Can you work these out from the model? Positions are in its coordinate system, mm. A direction names the side the tool comes from. Give positions to 0.01 mm unless a question says otherwise; leave off trailing zeros. Order: outer loops, then holes, each group sorted by start corner. A loop starts at its lowest first (then second) coordinate and runs counter-clockwise, first axis right, second up.
Item 1: If we mould it in two halves opening along X, with no side actions, what happens to faces 1 (the flat face through (17, 22, -10)), 2 (the cylindrical face through (-7.35, 5.1, -12.31)), 3 (the cylindrical face through (24.765, 5.028, 4.975))? For each: +X half, -X half, draft (parallel to the pull), parting line (faces both ways), or undercut.
Item 2: I want a section at A-A, the plane y = 16.75. Write out the boundary of the cut face in (x, z), then the cut area to 3 significant figures.
Item 3: I'm going to push flat-ended pins straight in: pin 1 Ø2 at (x, z) = (16, -2.5) entering from +Y; pin 2 Ø5 at (x, y) = (-6, 6.5) entering from +Z; pin 3 Ø3.5 at (y, z) = (2, 5) entering from -X. Where does each tip first touch, or does it pass through?
Item 4: If I drill on line 1 along Y through (x, z) = (-26, -17); line 2 along X through (y, z) = (8.5, 20.5); line 3 along Y through (x, z) = (6, 16), over which ranges is the centre line in solid material (lowest first)?
Item 5: Which directions (+Z, -Z, +X, -X, +Y, -Y) give clear straight access to the entire face, cutting with the end or side of a thin tool? Please do faces 4 (the flat face through (-7, 2, -13.169)), 5 (the flat face through (0, 5, -18.829)), 6 (the cylindrical face through (2.94, 15.92, 9.35)).
```python
from build123d import *

# Parameters (mm, degrees)
SALIENTE_EXTRUIR1_DEPTH    = 10
CROQUIS2_R                 = 2.5
CORTAR_EXTRUIR1_DEPTH      = 10
CROQUIS3_R                 = 9.8
SALIENTE_EXTRUIR2_DEPTH    = 12
CROQUIS4_W                 = 17.653456823
CROQUIS4_H                 = 4
CORTAR_EXTRUIR2_DEPTH      = 11.5
CORTAR_EXTRUIR3_DEPTH      = 62.373730343
CORTAR_EXTRUIR3_DEPTH_BACK = 62.373730343
CROQUIS5_W                 = 3.232473087
CROQUIS5_H                 = 4
REDONDEO1_R                = 1
REDONDEO2_R                = 5
MATRIZC7_COUNT             = 5
REDONDEO3_R                = 1
REDONDEO4_R                = 5
CORTAR_EXTRUIR4_DEPTH      = 54.438308108
CORTAR_EXTRUIR4_DEPTH_BACK = 6
CROQUIS7_W                 = 6.922650149
CROQUIS7_H                 = 26.338104106
REDONDEO5_R                = 3
CROQUIS9_R                 = 2.5
CORTAR_EXTRUIR5_DEPTH      = 22
CROQUIS10_R                = 2.5
SALIENTE_EXTRUIR3_DEPTH    = 12


with BuildPart() as part:
    # Croquis1 → Saliente-Extruir1 (new body)
    with BuildSketch(Plane(origin=(0, 0, 0), x_dir=(1, 0, 0), z_dir=(0, 1, 0))):
        with BuildLine():
            ThreePointArc((11.567553172, 25.331412183), (0, 35), (-11.567553172, 25.331412183))
            ThreePointArc((-11.567553172, 25.331412183), (-14.736015149, 20.282384831), (-20.51703411, 18.829233678))
            ThreePointArc((-20.51703411, 18.829233678), (-33.28697807, 10.815594803), (-27.666175138, -3.173559966))
            ThreePointArc((-27.666175138, -3.173559966), (-23.843373369, -7.747181632), (-24.247777601, -13.694305788))
            ThreePointArc((-24.247777601, -13.694305788), (-20.57248383, -28.315594803), (-5.531083401, -27.292780108))
            ThreePointArc((-5.531083401, -27.292780108), (0, -25.070406396), (5.531083401, -27.292780108))
            ThreePointArc((5.531083401, -27.292780108), (20.57248383, -28.315594803), (24.247777601, -13.694305788))
            ThreePointArc((24.247777601, -13.694305788), (23.843373369, -7.747181632), (27.666175138, -3.173559966))
            ThreePointArc((27.666175138, -3.173559966), (33.28697807, 10.815594803), (20.51703411, 18.829233678))
            ThreePointArc((20.51703411, 18.829233678), (14.736015149, 20.282384831), (11.567553172, 25.331412183))
        make_face()
    extrude(amount=SALIENTE_EXTRUIR1_DEPTH)

    # Croquis2 → Cortar-Extruir1 (cut)
    with BuildSketch(Plane(origin=(0, 10, 0), x_dir=(1, 0, 0), z_dir=(0, 1, 0))):
        with Locations(Location((-22.108224643, 7.183397635, 0), (0, 0, 270))):
            Circle(CROQUIS2_R)
        with Locations(Location((0, 23.245963057, 0), (0, 0, 270))):
            Circle(CROQUIS2_R)
        with Locations(Location((22.108224643, 7.183397635, 0), (0, 0, 270))):
            Circle(CROQUIS2_R)
        with Locations(Location((13.66363426, -18.806379164, 0), (0, 0, 270))):
            Circle(CROQUIS2_R)
        with Locations(Location((-13.66363426, -18.806379164, 0), (0, 0, 270))):
            Circle(CROQUIS2_R)
    extrude(amount=-CORTAR_EXTRUIR1_DEPTH, mode=Mode.SUBTRACT)

    # Croquis3 → Saliente-Extruir2 (add)
    with BuildSketch(Plane(origin=(0, 10, 0), x_dir=(1, 0, 0), z_dir=(0, 1, 0))):
        with Locations(Location((0, 0, 0), (0, 0, 270))):
            Circle(CROQUIS3_R)
    extrude(amount=SALIENTE_EXTRUIR2_DEPTH)

    # Croquis4 → Cortar-Extruir2 (cut, symmetric)
    with BuildSketch(Plane(origin=(0, 0, 0), x_dir=(0, 0, -1), z_dir=(1, 0, 0))):
        with Locations((27.65596209, 5)):
            Rectangle(CROQUIS4_W, CROQUIS4_H)
    cortar_extruir2 = extrude(amount=CORTAR_EXTRUIR2_DEPTH, both=True, mode=Mode.SUBTRACT)

    # Croquis5 → Cortar-Extruir3 (cut, two sides: drawn at the far end of the back side and taken through both)
    with BuildSketch(Plane.ZY.offset(-11.5).offset(-CORTAR_EXTRUIR3_DEPTH_BACK)):
        with Locations((-24.060237665, 5)):
            Rectangle(CROQUIS5_W, CROQUIS5_H)
    extrude(amount=CORTAR_EXTRUIR3_DEPTH + CORTAR_EXTRUIR3_DEPTH_BACK, mode=Mode.SUBTRACT)

    # Redondeo1
    # the kernel refuses this fillet: 1 mm, written as the material it takes off along each edge
    with BuildSketch(Plane(origin=(11.5, 3, -22.444001121), x_dir=(1, 0, 0), z_dir=(0, 1, 0)), Plane(origin=(-11.5, 3, -22.444001121), x_dir=(0, 0, 1), z_dir=(0, 1, 0))) as redondeo1_piece_1:
        with BuildLine():
            CenterArc((REDONDEO1_R, -REDONDEO1_R), REDONDEO1_R, 90, 90)
            Line((0, -REDONDEO1_R), (0, 0))
            Line((0, 0), (REDONDEO1_R, 0))
        make_face()
    extrude(amount=4, mode=Mode.SUBTRACT)
    with BuildSketch(Plane(origin=(12.699385644, 7, -22.444001121), x_dir=(-1, 0, 0), z_dir=(0, -1, 0))) as redondeo1_piece_2:
        with BuildLine():
            CenterArc((0.526987375, -1), REDONDEO1_R, 90, 53.849058394)
            ThreePointArc((-0.280478336, -0.410085493), (-0.137052587, -0.207222212), (0, 0))
            Line((0, 0), (0.526987375, 0))
        make_face()
    extrude(amount=4, mode=Mode.SUBTRACT)
    with BuildSketch(Plane(origin=(-12.699385644, 7, -22.444001121), x_dir=(1, 0, 0), z_dir=(0, -1, 0))) as redondeo1_piece_3:
        with BuildLine():
            CenterArc((0.526987375, 1), REDONDEO1_R, 216.150941606, 53.849058394)
            ThreePointArc((-0.280478336, 0.410085493), (-0.137052587, 0.207222212), (0, 0))
            Line((0, 0), (0.526987375, 0))
        make_face()
    extrude(amount=4, mode=Mode.SUBTRACT)

    # Redondeo2
    redondeo2_edges = [part.edges().sort_by_distance(p)[0] for p in [
        (-11.5, 5, -18.829233678),
        (11.5, 5, -18.829233678),
    ]]
    fillet(redondeo2_edges, radius=REDONDEO2_R)

    # MatrizC7: Cortar-Extruir2 ×5 about axis
    matrizc7_axis = Axis((0, 0, 0), (0, 1, 0))
    for i in range(1, MATRIZC7_COUNT):
        add(cortar_extruir2.rotate(matrizc7_axis, i * 360 / MATRIZC7_COUNT), mode=Mode.SUBTRACT)

    # Redondeo3
    # the kernel refuses this fillet: 1 mm, written as the material it takes off along each edge
    with BuildSketch(Plane(origin=(27.973473546, 7, 3.002683051), x_dir=(-0.745583502081635, 0, 0.6664122158421801), z_dir=(0, -1, 0)), Plane(origin=(5.788557435, 7, 27.532234391), x_dir=(-0.864193653284182, 0, -0.5031593481426527), z_dir=(0, -1, 0)), Plane(origin=(-24.395948306, 7, 14.013173589), x_dir=(0.21148245149008985, 0, -0.9773817947515403), z_dir=(0, -1, 0)), Plane(origin=(-20.866082676, 7, -18.871616823), x_dir=(0.9948969963292142, 0, -0.10089582099922498), z_dir=(0, -1, 0))) as redondeo3_piece_1:
        with BuildLine():
            CenterArc((4.661949033, 0.96239971), REDONDEO3_R, 113.790758155, 140.447525624)
            Line((4.258551325, 1.877424458), (4.218211554, 1.968926933))
            Line((4.218211554, 1.968926933), (-0.040339771, 0.091502475))
            Line((-0.040339771, 0.091502475), (0.020546947, -0.097866353))
            ThreePointArc((0.020546947, -0.097866353), (0.366456105, -0.019823583), (4.363148054, -0.096239971))
            Line((4.363148054, -0.096239971), (4.390311779, 0))
        make_face()
    extrude(amount=4, mode=Mode.SUBTRACT)
    with BuildSketch(Plane(origin=(20.866082676, 7, -18.871616823), x_dir=(-0.9948969963292025, 0, -0.10089582099933926), z_dir=(0, -1, 0)), Plane(origin=(24.395948306, 7, 14.013173589), x_dir=(-0.2114824514899068, 0, -0.9773817947515798), z_dir=(0, -1, 0)), Plane(origin=(-5.788557435, 7, 27.532234391), x_dir=(0.8641936532842898, 0, -0.5031593481424677), z_dir=(0, -1, 0)), Plane(origin=(-27.973473546, 7, 3.002683051), x_dir=(0.7455835020815682, 0, 0.666412215842255), z_dir=(0, -1, 0))) as redondeo3_piece_2:
        with BuildLine():
            CenterArc((4.661949033, -0.96239971), REDONDEO3_R, 105.761716221, 140.447525624)
            Line((4.258551325, -1.877424458), (4.218211554, -1.968926933))
            Line((4.218211554, -1.968926933), (-0.040339771, -0.091502475))
            Line((-0.040339771, -0.091502475), (0.020546947, 0.097866353))
            ThreePointArc((0.020546947, 0.097866353), (0.366456105, 0.019823583), (4.363148054, 0.096239971))
            Line((4.363148054, 0.096239971), (4.390311779, 0))
        make_face()
    extrude(amount=4, mode=Mode.SUBTRACT)

    # Redondeo4
    redondeo4_edges = [part.edges().sort_by_distance(p)[0] for p in [
        (14.353969951, 5, -16.755703135),
        (21.461360822, 5, 5.11859674),
        (20.371241303, 5, 8.473639636),
        (1.763850433, 5, 21.992700438),
        (-1.763850433, 5, 21.992700438),
        (-20.371241303, 5, 8.473639636),
        (-21.461360822, 5, 5.11859674),
        (-14.353969951, 5, -16.755703135),
    ]]
    fillet(redondeo4_edges, radius=REDONDEO4_R)

    # Croquis7 → Cortar-Extruir4 (cut, two sides: drawn at the far end of the back side and taken through both)
    with BuildSketch(Plane.XZ.offset(-CORTAR_EXTRUIR4_DEPTH_BACK)):
        with Locations((-6.630731168, 0)):
            Rectangle(CROQUIS7_W, CROQUIS7_H)
        with Locations((7.131163709, 0)):
            Rectangle(CROQUIS7_W, CROQUIS7_H)
    extrude(amount=CORTAR_EXTRUIR4_DEPTH + CORTAR_EXTRUIR4_DEPTH_BACK, mode=Mode.SUBTRACT)

    # Redondeo5
    redondeo5_edges = [part.edges().sort_by_distance(p)[0] for p in [
        (-6.630731167, 6, -13.169052053),
        (-3.169406093, 6, 0),
        (-6.630731167, 6, 13.169052053),
        (3.669838634, 6, 0),
        (7.131163708, 6, -13.169052053),
        (7.131163708, 6, 13.169052053),
    ]]
    fillet(redondeo5_edges, radius=REDONDEO5_R)

    # Croquis9 → Cortar-Extruir5 (cut)
    with BuildSketch(Plane(origin=(0, 22, 0), x_dir=(1, 0, 0), z_dir=(0, 1, 0))):
        with Locations(Location((17.5, 0, 0), (0, 0, 270))):
            Circle(CROQUIS9_R)
        with Locations(Location((-17.5, 0, 0), (0, 0, 270))):
            Circle(CROQUIS9_R)
    extrude(amount=-CORTAR_EXTRUIR5_DEPTH, mode=Mode.SUBTRACT)

    # Croquis10 → Saliente-Extruir3 (add)
    with BuildSketch(Plane(origin=(0, 10, 0), x_dir=(1, 0, 0), z_dir=(0, 1, 0))):
        with Locations(Location((17.320508076, 10, 0), (0, 0, 270))):
            Circle(CROQUIS10_R)
        with Locations(Location((-17.320508076, -10, 0), (0, 0, 270))):
            Circle(CROQUIS10_R)
    extrude(amount=SALIENTE_EXTRUIR3_DEPTH)


solid = part.part
```
Results list:
1. face 1: draft
1. face 2: undercut
1. face 3: +X half
2. outline: circle Ø5 at (-17.32, 10); circle Ø19.6 at (0, 0); circle Ø5 at (17.32, -10)
2. area: 341 mm2
3. pin 1: stops at y = 10
3. pin 2: stops at z = 29.34
3. pin 3: stops at x = -27.53
4. line 1: y = 0 to 3, 7 to 10
4. line 2: x = -25.3 to -15.5, -11.82 to 11.82, 15.5 to 25.3
4. line 3: y = 0 to 10
5. face 4: -Y
5. face 5: -Z
5. face 6: +Y
